from build123d import *

# Parameters (mm, degrees)
SKETCH1_R           = 20.25
BOSS_EXTRUDE1_DEPTH = 9
SKETCH2_R           = 17.75
CUT_EXTRUDE1_DEPTH  = 8
CIRPATTERN1_COUNT   = 3
SKETCH5_R           = 1.5
CUT_EXTRUDE2_DEPTH  = 8
CIRPATTERN2_COUNT   = 3


with BuildPart() as part:
    # Sketch1 → Boss-Extrude1 (new body)
    with BuildSketch(Plane(origin=(0, 0, 0), x_dir=(1, 0, 0), z_dir=(0, 1, 0))):
        with Locations(Location((0, 0, 0), (0, 0, 270))):
            Circle(SKETCH1_R)
    extrude(amount=BOSS_EXTRUDE1_DEPTH)

    # Sketch2 → Cut-Extrude1 (cut)
    with BuildSketch(Plane(origin=(0, 9, 0), x_dir=(1, 0, 0), z_dir=(0, 1, 0))):
        with Locations(Location((0, 0, 0), (0, 0, 270))):
            Circle(SKETCH2_R)
    extrude(amount=-CUT_EXTRUDE1_DEPTH, mode=Mode.SUBTRACT)

    # Sketch4 → CSK SLOT for M2 Countersunk Flat Head Screw1 (revolve, cut)
    with BuildSketch(Plane(origin=(11.609715894, 0, 11.00974554), x_dir=(0, 0, -1), z_dir=(1, 0, 0))):
        Polygon((0, 0), (0, 6.521032743), (1.2, 5.8), (1.2, 1), (2.2, 0), align=None)
    csk_slot_for_m2_countersunk_flat_head_sc = revolve(axis=Axis((11.609715894, -6.35, 11.00974554), (0, 1, 0)), mode=Mode.SUBTRACT)

    # CirPattern1: CSK SLOT for M2 Countersunk Flat Head Screw1 ×3 about axis
    cirpattern1_axis = Axis((0, 0, 0), (0, 1, 0))
    for i in range(1, CIRPATTERN1_COUNT):
        add(csk_slot_for_m2_countersunk_flat_head_sc.rotate(cirpattern1_axis, i * 360 / CIRPATTERN1_COUNT), mode=Mode.SUBTRACT)

    # Sketch5 → Cut-Extrude2 (cut)
    with BuildSketch(Plane.XZ):
        with Locations(Location((0, 0, 0), (0, 0, 270))):
            Circle(SKETCH5_R)
    extrude(amount=-CUT_EXTRUDE2_DEPTH, mode=Mode.SUBTRACT)

    # Sketch6 → M2 Tapped Hole1 (revolve, cut)
    with BuildSketch(Plane(origin=(-4.560794248, 4.445790719, 19.729715047), x_dir=(0.974306915892993, 0, 0.22522440729877435), z_dir=(0, 1, 0))):
        Polygon((0, 0), (0, 4.980688495), (0.8, 4.5), (0.8, 0), align=None)
    m2_tapped_hole1 = revolve(axis=Axis((-5.990969234, 4.445790719, 25.916563963), (0.22522440729877433, 0, -0.9743069158929931)), mode=Mode.SUBTRACT)

    # CirPattern2: M2 Tapped Hole1 ×3 about axis
    cirpattern2_axis = Axis((0, 9, 0), (0, -1, 0))
    for i in range(1, CIRPATTERN2_COUNT):
        add(m2_tapped_hole1.rotate(cirpattern2_axis, i * 360 / CIRPATTERN2_COUNT), mode=Mode.SUBTRACT)


solid = part.part
CAD build for the part. Positions are in the model's coordinates, mm. A direction names the side the tool comes from. Coordinates: 2 decimals unless noted, no trailing zeros. Order: outer loops, then holes, each group sorted by start corner. A loop starts at its lowest first (then second) coordinate and runs counter-clockwise, first axis right, second up.
Item 1: Pin check, flat tips, straight feed: pin 1 Ø3 at (y, z) = (3.5, 0.5) entering from +X; pin 2 Ø2 at (y, z) = (4, 0) entering from -X; pin 3 Ø1 at (x, y) = (3, 4.5) entering from -Z; pin 4 Ø1.8 at (x, z) = (0, 0) entering from +Y. Stop position of each tip, or through.
Check sheet entries:
pin 1: stops at x = 20.25
pin 2: stops at x = -20.25
pin 3: stops at z = -20.1
pin 4: passes through
Item 2: 3-axis set-ups, long thin cutter, end or side, ignore diameter. For faces 5 (the face through (-15.747, 5.056, 8.191)), 6 (the face through (17, 4, 11)): which of +Z, -Z, +X, -X, +Y, -Y reach the whole face in a straight line?
Check sheet entries:
face 5: +Y
face 6: +Y, -Y
Item 3: Band-saw the part on D-D on y = 2. List the corners of the cut face in (x, z).
Check sheet entries:
outline: circle Ø40.5 at (0, 0); hole circle Ø35.5 at (0, 0)
Item 4: Two-plate mould, pull along Y, no slides. Class faces 1 (the face through (18.23, 5.227, -5.387)), 2 (the face through (0, 0, 4)), 3 (the face through (-4.45, 5.227, 18.481)), 4 (the face through (-4, 1, 0)): +Y half, -Y half, draft (parallel to the pull), parting line (faces both ways), or undercut.
Check sheet entries:
face 1: undercut
face 2: -Y half
face 3: undercut
face 4: +Y half
Item 5: Band-saw the part on C-C on x = 7.5. List the corners of the cut face in (y, z).
Check sheet entries:
outline: (0, -18.81) - (9, -18.81) - (9, -16.09) - (1, -16.09) - (1, 16.09) - (9, 16.09) - (9, 18.81) - (0, 18.81) - close
Item 6: Band-saw the part on B-B on x = 0. List the corners of the cut face in (y, z).
Check sheet entries:
outline: (0, -20.25) - (9, -20.25) - (9, -17.75) - (1, -17.75) - (1, -1.5) - (0, -1.5) - close; (0, 1.5) - (1, 1.5) - (1, 17.75) - (9, 17.75) - (9, 20.25) - (0, 20.25) - close
Item 7: Band-saw the part on A-A on z = 0. List the corners of the cut face in (x, y), plus the area to 3 significant figures.
Check sheet entries:
outline: (-20.25, 0) - (-1.5, 0) - (-1.5, 1) - (-17.75, 1) - (-17.75, 9) - (-20.25, 9) - close; (1.5, 0) - (20.25, 0) - (20.25, 9) - (17.75, 9) - (17.75, 1) - (1.5, 1) - close
area: 77.5 mm2
Item 8: Drill centre lines: L1, parallel to X at y = 0.6, z = 0; L2, parallel to X at y = 3.25, z = 0; L3, parallel to Y at x = -7, z = 12.5. Where is each one in solid material? Low to high.
Check sheet entries:
L1: x = -20.25 to -1.5, 1.5 to 20.25
L2: x = -20.25 to -17.75, 17.75 to 20.25
L3: y = 0 to 1
